Geometry check sheet. Reference: the model listing, model coordinates, mm. A direction names the side the tool comes from. Coordinates: 2 decimals unless noted, no trailing zeros. Loops run counter-clockwise (first coordinate to the right, second up) from the corner with the lowest first, then second, coordinate; pieces in that order, holes last.
from build123d import *

# Parameters (mm, degrees)
F1_DEPTH = 3
F2_DEPTH = 7


with BuildPart() as f1:
    # F0 (on Top) → F1 (new body)
    with BuildSketch(Plane.XY):
        Polygon((-13.49, 7.788455), (-13.49, -7.788455), (0, -15.57691), (13.49, -7.788455), (13.49, 7.788455), (0, 15.57691), align=None)
        Polygon((0, 12.112809), (10.49, 6.056404), (10.49, -6.056404), (0, -12.112809), (-10.49, -6.056404), (-10.49, 6.056404), align=None, mode=Mode.SUBTRACT)
        Polygon((10.49, -6.056404), (10.49, 6.056404), (0, 12.112809), (-10.49, 6.056404), (-10.49, -6.056404), (0, -12.112809), align=None)
    extrude(amount=F1_DEPTH)

    # F0 (on Top) → F2 (join)
    with BuildSketch(Plane.XY):
        Polygon((-13.49, 7.788455), (-13.49, -7.788455), (0, -15.57691), (13.49, -7.788455), (13.49, 7.788455), (0, 15.57691), align=None)
        Polygon((0, 12.112809), (10.49, 6.056404), (10.49, -6.056404), (0, -12.112809), (-10.49, -6.056404), (-10.49, 6.056404), align=None, mode=Mode.SUBTRACT)
    extrude(amount=F2_DEPTH)


solid = f1.part
(1) Sectioned sample at A-A on z = 1.75. Record the cut outline in (x, y), and give its area (3 significant figures).
Findings:
outline: (-13.49, -7.79) - (0, -15.58) - (13.49, -7.79) - (13.49, 7.79) - (0, 15.58) - (-13.49, 7.79) - close
area: 630 mm2
(2) Gauge pin test, flat end, axial feed: pin 1 Ø2 at (x, z) = (-9, 4) entering from +Y. Record the tip position at first contact, or that the pin passes through.
Findings:
pin 1: stops at y = 10.96
(3) Sectioned sample at C-C on z = 5.75. Record the cut outline in (x, y), and give its area (3 significant figures).
Findings:
outline: (-13.49, -7.79) - (0, -15.58) - (13.49, -7.79) - (13.49, 7.79) - (0, 15.58) - (-13.49, 7.79) - close; hole (-10.49, -6.06) - (0, -12.11) - (10.49, -6.06) - (10.49, 6.06) - (0, 12.11) - (-10.49, 6.06) - close
area: 249 mm2
(4) Scan lines: L1, parallel to X at y = 1.5, z = 4; L2, parallel to Z at x = 3, y = -3.5; L3, parallel to Y at x = -3.5, z = 6.25. Record each from-to range of solid material in increasing order.
Findings:
L1: x = -13.49 to -10.49, 10.49 to 13.49
L2: z = 0 to 3
L3: y = -13.56 to -10.09, 10.09 to 13.56
(5) Sectioned sample at B-B on y = 5. Record the cut outline in (x, z).
Findings:
outline: (-13.49, 0) - (13.49, 0) - (13.49, 7) - (10.49, 7) - (10.49, 3) - (-10.49, 3) - (-10.49, 7) - (-13.49, 7) - close
(6) Sectioned sample at D-D on x = -6.25. Record the cut outline in (y, z), and give its area (3 significant figures).
Findings:
outline: (-11.97, 0) - (11.97, 0) - (11.97, 7) - (8.5, 7) - (8.5, 3) - (-8.5, 3) - (-8.5, 7) - (-11.97, 7) - close
area: 99.5 mm2
(7) Draft check along X on faces 3 (the flat face through (5.17, 9.13, 4.97)), 4 (the flat face through (0, 0, 0)), 5 (the flat face through (-6.651, 11.737, 3.451)). Enter one of: +X half, -X half, draft (parallel to the pull), parting line (faces both ways), or undercut.
Findings:
face 3: undercut
face 4: draft
face 5: -X half
(8) Access from +Z, -Z, +X, -X, +Y, -Y to the whole of each face (thin tool, end or side, straight path). Record for faces 1 (the flat face through (10.49, 0, 5)), 2 (the flat face through (-5, -10, 7)).
Findings:
face 1: +Z
face 2: +Z, +X, -X, +Y, -Y
